Answer from the drawing. Dimensions are ordinates in mm from the lowest x, y and z of the part. Give positions to 0.01 mm unless a question says otherwise; leave off trailing zeros. Loops run counter-clockwise (first coordinate to the right, second up) from the corner with the lowest first, then second, coordinate; pieces in that order, holes last.
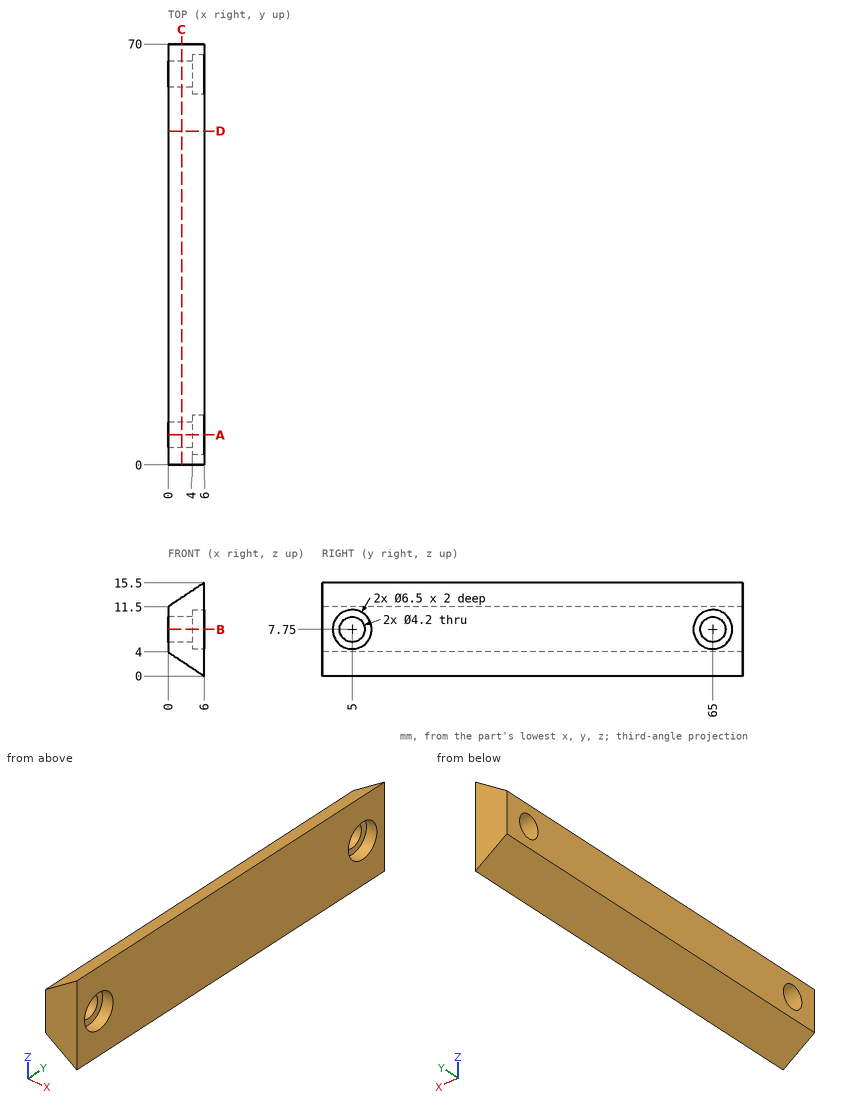
Item 1: Find section B-B, the plane z = 7.75. Write down the section's boundary in (x, y).
Item 2: Consider line 1 (X direction, y = 3.5, z = 1); line 2 (Y direction, x = 4.4, z = 5.25); line 3 (Z direction, x = 4.9, y = 5). Determine where each line is inside the solid, lowest interval first.
Item 3: Find section A-A, the plane y = 5. Write down the section's boundary in (x, z).
Item 4: Find section C-C, the plane x = 2.25. Write down the section's boundary in (y, z), plus the area to 3 significant figures.
Item 5: Find section D-D, the plane y = 55.5. Write down the section's boundary in (x, z).
Item 6: Flat-ended cylindrical pins translate along their axes: pin 1 Ø6 at (y, z) = (65, 7.75) entering from +X; pin 2 Ø1 at (x, y) = (3, 51.5) entering from +Z. Find the tip coordinate at first contact, or state that the pin passes through.
Ans:
1. outline: (0, 0) - (6, 0) - (6, 1.75) - (4, 1.75) - (4, 2.9) - (0, 2.9) - close; (0, 7.1) - (4, 7.1) - (4, 8.25) - (6, 8.25) - (6, 61.75) - (4, 61.75) - (4, 62.9) - (0, 62.9) - close; (0, 67.1) - (4, 67.1) - (4, 68.25) - (6, 68.25) - (6, 70) - (0, 70) - close
2. line 1: x = 4.5 to 6
2. line 2: y = 0 to 2.92, 7.08 to 62.92, 67.08 to 70
2. line 3: z = 0.73 to 4.5, 11 to 14.77
3. outline: (0, 4) - (6, 0) - (6, 4.5) - (4, 4.5) - (4, 5.65) - (0, 5.65) - close; (0, 9.85) - (4, 9.85) - (4, 11) - (6, 11) - (6, 15.5) - (0, 11.5) - close
4. outline: (0, 2.5) - (70, 2.5) - (70, 13) - (0, 13) - close; hole circle Ø4.2 at (5, 7.75); hole circle Ø4.2 at (65, 7.75)
4. area: 707 mm2
5. outline: (0, 4) - (6, 0) - (6, 15.5) - (0, 11.5) - close
6. pin 1: stops at x = 4
6. pin 2: stops at z = 13.83
